from build123d import *

# Parameters (mm, degrees)
F0_R     = 47.5
F1_DEPTH = 2
F1_TAPER = -30
F2_R     = 42.5
F2_R_2   = 40
F3_DEPTH = 10
F5_DEPTH = 25
F6_DEPTH = 3


with BuildPart() as f1:
    # F0 (on Front) → F1 (new body)
    with BuildSketch(Plane.XZ):
        Circle(F0_R)
    extrude(amount=-F1_DEPTH, taper=F1_TAPER)

    # F2 (on face) → F3 (join)
    with BuildSketch(Plane(origin=(0, 2, 0), x_dir=(-1, 0, 0), z_dir=(0, 1, 0))):
        Circle(F2_R)
        Circle(F2_R_2, mode=Mode.SUBTRACT)
    extrude(amount=F3_DEPTH)

    # F4 (on face) → F5 (cut)
    with BuildSketch(Plane(origin=(0, 2, 0), x_dir=(-1, 0, 0), z_dir=(0, 1, 0))):
        with BuildLine():
            ThreePointArc((20.9875792028, 29.753044393), (7.9449809873, 18.8289116609), (2.3533185627, 2.7609511341))
            ThreePointArc((2.3533185627, 2.7609511341), (15.0280319463, 13.9390568271), (20.9875792028, 29.753044393))
        make_face()
        with BuildLine():
            ThreePointArc((34.4677089509, 11.7345290116), (17.4949812297, 10.5629668651), (3.5267210693, 0.8504104431))
            ThreePointArc((3.5267210693, 0.8504104431), (20.3511052704, 2.4436783097), (34.4677089509, 11.7345290116))
        make_face()
        with BuildLine():
            ThreePointArc((34.7823453941, -10.7661776103), (20.3624932749, -1.7376722511), (3.3530359963, -1.3849581328))
            ThreePointArc((3.3530359963, -1.3849581328), (17.9007480898, -9.9851022645), (34.7823453941, -10.7661776103))
        make_face()
        with BuildLine():
            ThreePointArc((21.8113081051, -29.1545703139), (15.4522249847, -13.3745796286), (1.8986051383, -3.091319775))
            ThreePointArc((1.8986051383, -3.091319775), (8.612913563, -18.5999131547), (21.8113081051, -29.1545703139))
        make_face()
        with BuildLine():
            ThreePointArc((0.5090924591, -36.4069080851), (4.6397319522, -19.9028521733), (-0.2810283514, -3.6169023332))
            ThreePointArc((-0.2810283514, -3.6169023332), (-3.9647612027, -20.1101894077), (0.5090924591, -36.4069080851))
        make_face()
        with BuildLine():
            ThreePointArc((-20.9875792028, -29.753044393), (-7.9449809873, -18.8289116609), (-2.3533185627, -2.7609511341))
            ThreePointArc((-2.3533185627, -2.7609511341), (-15.0280319463, -13.9390568271), (-20.9875792028, -29.753044393))
        make_face()
        with BuildLine():
            ThreePointArc((-34.4677089509, -11.7345290116), (-17.4949812297, -10.5629668651), (-3.5267210693, -0.8504104431))
            ThreePointArc((-3.5267210693, -0.8504104431), (-20.3511052704, -2.4436783097), (-34.4677089509, -11.7345290116))
        make_face()
        with BuildLine():
            ThreePointArc((-21.8113081051, 29.1545703139), (-15.4522249847, 13.3745796286), (-1.8986051383, 3.091319775))
            ThreePointArc((-1.8986051383, 3.091319775), (-8.612913563, 18.5999131547), (-21.8113081051, 29.1545703139))
        make_face()
        with BuildLine():
            ThreePointArc((-0.5090924591, 36.4069080851), (-4.6397319522, 19.9028521733), (0.2810283514, 3.6169023332))
            ThreePointArc((0.2810283514, 3.6169023332), (3.9647612027, 20.1101894077), (-0.5090924591, 36.4069080851))
        make_face()
        with BuildLine():
            ThreePointArc((-34.7823453941, 10.7661776103), (-20.3624932749, 1.7376722511), (-3.3530359963, 1.3849581328))
            ThreePointArc((-3.3530359963, 1.3849581328), (-17.9007480898, 9.9851022645), (-34.7823453941, 10.7661776103))
        make_face()
    extrude(amount=-F5_DEPTH, mode=Mode.SUBTRACT)

    # F6 (add): a face of the model
    f6_faces = [f1.faces().sort_by_distance(p)[0] for p in [
        (0, 2, 0),
    ]]
    extrude(f6_faces, amount=F6_DEPTH)


solid = f1.part
Geometry: final body of the model. Coordinates: model frame, mm. A direction names the side the tool comes from. Round coordinates to 2 decimals unless told otherwise and drop trailing zeros. Write item = value, one per line.
Item 1: Section query A-A on x = 13. State how many separate pieces and enclosed holes the cut face has, then the cut area to 3 significant figures.
Findings:
separate_pieces = 5
enclosed_holes = 0
area = 257 mm^2
Item 2: Material intervals for line 1 along Z through (x, y) = (0, 9.25); line 2 along Z through (x, y) = (24.5, 1.75); line 3 along Y through (x, z) = (-15.5, 14), sorted ascending. Write a range as [from, to].
Findings:
line_1 = [-42.5, -40], [40, 42.5]
line_2 = [-41.87, -12.17], [-4.21, 3.29], [11.28, 41.87]
line_3 = [0, 5]
Item 3: Access query for faces 1 (the face through (29, 12, -28)), 2 (the face through (8.67, 8.45, -39.05)). Directions: +Z, -Z, +X, -X, +Y, -Y. A direction counts if a zero-diameter tool reaches every point of the face in a straight line with its end or side. Return the directions, or none.
Findings:
face_1 = +Z, -Z, +X, -X, +Y
face_2 = +Y
Item 4: Pin query (flat end, axial travel): P1, Ø4, axis at x = -29.5, y = 2.5, coming from the +Z side; P2, Ø1.5, axis at x = -36, z = 4, coming from the +Y side; P3, Ø1, axis at x = -20.5, y = 6, coming from the -Z side. Return the tip coordinate at first contact, or that it passes through.
Findings:
P1 = 40.09
P2 = 5
P3 = -37.5
Item 5: Pull-direction query (Z, two-part tool) for faces 3 (the face through (15.6, 2.46, 13.57)), 4 (the face through (0, 2, -43)), 5 (the face through (33.727, 6.93, -25.861)); classes: pulls with the +Z half, pulls with the -Z half, needs draft (parallel to the pull), parting line crosses it, or undercut.
Findings:
face_3 = undercut
face_4 = needs draft
face_5 = parting line crosses it
